from build123d import *

# Parameters (mm, degrees)
F0_R      = 13.5
F1_DEPTH  = 3
F2_R      = 5
F2_R_2    = 3.85
F3_DEPTH  = 1.3
F3_FACE_R = 3.85
F4_DEPTH  = 3.3


with BuildPart() as f1:
    # F0 (on Top) → F1 (new body)
    with BuildSketch(Plane.XY):
        Circle(F0_R)
    extrude(amount=F1_DEPTH)

    # F2 (on Top) → F3 (join)
    with BuildSketch(Plane.XY):
        Circle(F2_R)
        Circle(F2_R_2, mode=Mode.SUBTRACT)
    extrude(amount=-F3_DEPTH)

    # F3_face (on face) → F4 (join)
    with BuildSketch(Plane(origin=(0, 0, 0), x_dir=(1, 0, 0), z_dir=(0, 0, -1))):
        Circle(F3_FACE_R)
    extrude(amount=F4_DEPTH)


solid = f1.part
Design review of the part built by this model. Coordinates are the model's own, in mm. A direction names the side the tool comes from. Round coordinates to 2 decimals unless told otherwise and drop trailing zeros. Order: outer loops, then holes, each group sorted by start corner. A loop starts at its lowest first (then second) coordinate and runs counter-clockwise, first axis right, second up.
1) Consider section C-C (z = -2.75). State the section outline as (x, y) points, plus the area to 3 significant figures.
The answers:
outline: circle Ø7.7 at (0, 0)
area: 46.6 mm2
2) Machinability: for faces 1 (the flat face through (0, 0, -3.3)), 2 (the cylindrical face through (-0.83, 3.76, -2.29)), which of the approach directions +Z, -Z, +X, -X, +Y, -Y give a long, thin tool a straight path to every point of the face, cutting with its end or side? Answer none if there is none.
The answers:
face 1: -Z, +X, -X, +Y, -Y
face 2: -Z
3) Consider section D-D (z = 1). State the section outline as (x, y) points.
The answers:
outline: circle Ø27 at (0, 0)
4) For L1, parallel to Z at x = -3.5, y = 9.75; L2, parallel to X at y = 0, z = -2.25; L3, parallel to Y at x = -0.25, z = -2.5, list the stretches that pass through material, from the lowest coordinate up.
The answers:
L1: z = 0 to 3
L2: x = -3.85 to 3.85
L3: y = -3.84 to 3.84
5) Clearance check with flat-ended pins moving along their axes: pin 1 Ø1 at (x, z) = (-4, 1.5) entering from -Y; pin 2 Ø2 at (x, y) = (-9.5, 2) entering from -Z. State where each tip first meets the part, or that it passes through.
The answers:
pin 1: stops at y = -13.04
pin 2: stops at z = 0
6) Consider section A-A (y = 0). State the section outline as (x, z) points.
The answers:
outline: (-13.5, 0) - (-5, 0) - (-5, -1.3) - (-3.85, -1.3) - (-3.85, -3.3) - (3.85, -3.3) - (3.85, -1.3) - (5, -1.3) - (5, 0) - (13.5, 0) - (13.5, 3) - (-13.5, 3) - close
7) Draft analysis for pull direction Y (two halves, no side actions). For faces 3 (the flat face through (0, 0, 3)), 4 (the cylindrical face through (-2.93, -13.18, 1.48)), state which applies: released by +Y, released by -Y, zero draft, split by the parting line, or undercut.
The answers:
face 3: zero draft
face 4: split by the parting line
